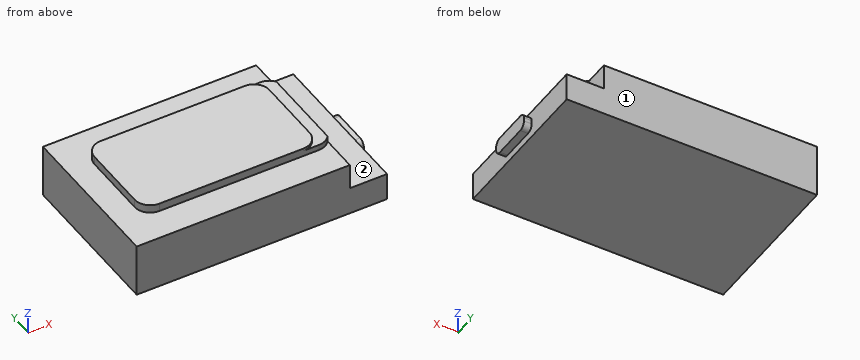
Solid Edge part; units mm, degrees
sketch "Sketch1" plane through (0, 0, 0) normal (0, 0, 1) x (1, 0, 0)
  line L0 (-25, -15.15) -> (25, -15.15)
  line L1 (25, -15.15) -> (25, 15.15)
  line L2 (25, 15.15) -> (-25, 15.15)
  line L3 (-25, 15.15) -> (-25, -15.15)
extrude "Protrusion1" add sketch "Sketch1" along normal blind 12
sketch "Sketch2" plane through (25, 0, 6) normal (1, 0, 0) x (0, 1, 0)
  line L0 (-0.65, -1.4) -> (2.65, -1.4)
  arc A0 (2.65, -1.4) -> (3.85, -2.6) centre (2.65, -2.6) cw
  line L1 (3.85, -2.6) -> (3.85, -3.3)
  arc A1 (2.65, -4.5) -> (3.85, -3.3) centre (2.65, -3.3) ccw
  line L2 (2.65, -4.5) -> (-3.95, -4.5)
  arc A2 (-5.15, -3.3) -> (-3.95, -4.5) centre (-3.95, -3.3) ccw
  line L3 (-5.15, -3.3) -> (-5.15, -2.6)
  arc A3 (-5.15, -2.6) -> (-3.95, -1.4) centre (-3.95, -2.6) cw
  line L4 (-3.95, -1.4) -> (-0.65, -1.4)
  line L5 (-15.15, -6) -> (15.15, -6)
  line L6 (15.15, -6) -> (15.15, 6)
  line L7 (15.15, 6) -> (-15.15, 6)
  line L8 (-15.15, 6) -> (-15.15, -6)
extrude "Wycięcie_1" cut sketch "Sketch2" against normal blind 1.5
sketch "Sketch3" plane through (-0.75, 0, 12) normal (0, 0, 1) x (1, 0, 0)
  line L0 (17.05, 15.15) -> (17.05, -15.15)
  line L1 (17.05, -15.15) -> (24.25, -15.15)
  line L2 (24.25, -15.15) -> (24.25, 15.15)
  line L3 (24.25, 15.15) -> (17.05, 15.15)
extrude "Wycięcie_2" cut sketch "Sketch3" against normal blind 6.6
sketch "Sketch4" plane through (-4.35, 0, 12) normal (0, 0, 1) x (1, 0, 0)
  line L0 (1.7674, -9.15) -> (-12.65, -9.15)
  arc A0 (-15.65, -6.15) -> (-12.65, -9.15) centre (-12.65, -6.15) ccw
  line L1 (-15.65, -6.15) -> (-15.65, 6.85)
  arc A1 (-15.65, 6.85) -> (-12.65, 9.85) centre (-12.65, 6.85) cw
  line L2 (-12.65, 9.85) -> (18.25, 9.85)
  arc A2 (18.25, 9.85) -> (21.25, 6.85) centre (18.25, 6.85) cw
  line L3 (21.25, 6.85) -> (21.25, -6.15)
  arc A3 (18.25, -9.15) -> (21.25, -6.15) centre (18.25, -6.15) ccw
  line L4 (18.25, -9.15) -> (1.7674, -9.15)
  line L5 (-28.1147, 19.5962) -> (36.8147, 19.5962)
  line L6 (36.8147, 19.5962) -> (36.8147, -19.5962)
  line L7 (36.8147, -19.5962) -> (-28.1147, -19.5962)
  line L8 (-28.1147, -19.5962) -> (-28.1147, 19.5962)
extrude "Wycięcie_3" cut sketch "Sketch4" against normal blind 1.6
sketch "Sketch5" plane through (-1.85, 0.35, 12) normal (0, 0, 1) x (1, 0, 0)
  line L0 (-18.15, 0) -> (-18.15, 6.5)
  arc A0 (-18.15, 6.5) -> (-15.15, 9.5) centre (-15.15, 6.5) cw
  line L1 (-15.15, 9.5) -> (12.75, 9.5)
  arc A1 (12.75, 9.5) -> (15.75, 6.5) centre (12.75, 6.5) cw
  line L2 (15.75, 6.5) -> (15.75, -6.5)
  arc A2 (15.75, -6.5) -> (12.75, -9.5) centre (12.75, -6.5) cw
  line L3 (-15.15, -9.5) -> (12.75, -9.5)
  arc A3 (-18.15, -6.5) -> (-15.15, -9.5) centre (-15.15, -6.5) ccw
  line L4 (-18.15, 0) -> (-18.15, -6.5)
  line L5 (-29.5576, 18.3934) -> (33.2576, 18.3934)
  line L6 (33.2576, 18.3934) -> (33.2576, -19.0934)
  line L7 (33.2576, -19.0934) -> (-29.5576, -19.0934)
  line L8 (-29.5576, -19.0934) -> (-29.5576, 18.3934)
extrude "Wycięcie_4" cut sketch "Sketch5" against normal blind 0.5
Source: CAD feature listing. Evaluate the final solid. Frame: model axes, mm. Face numbers are marked on the shaded views. A direction names the side the tool comes from. Coordinates: 2 decimals unless noted, no trailing zeros. Order: outer loops, then holes, each group sorted by start corner. A loop starts at its lowest first (then second) coordinate and runs counter-clockwise, first axis right, second up.
Item 1: Cut plane C-C (z = 6). Return loops of the section in (x, y), plus the area to 3 significant figures.
Output values:
outline: (-25, -15.15) - (16.3, -15.15) - (16.3, 15.15) - (-25, 15.15) - close
area: 1,250 mm2
Item 2: Material intervals for line 1 (Z direction, x = -13, y = -10.5); line 2 (Z direction, x = 18, y = -8); line 3 (X direction, y = 5.5, z = 5), sorted ascending.
Output values:
line 1: z = 0 to 10.4
line 2: z = 0 to 5.4
line 3: x = -25 to 23.5
Item 3: First-contact query: P1, Ø1, axis at y = -12, z = 10, coming from the +X side; P2, Ø0.8, axis at x = 24, z = 3, coming from the +Y side; P3, Ø0.8, axis at x = 24.5, y = -2, coming from the -Z side. Flat tips, straight axial feed; report the tip coordinate or a pass-through.
Output values:
P1: stops at x = 16.3
P2: stops at y = 3.85
P3: stops at z = 1.5
Item 4: Cut plane D-D (y = -11). Return loops of the section in (x, z), plus the area to 3 significant figures.
Output values:
outline: (-25, 0) - (23.5, 0) - (23.5, 5.4) - (16.3, 5.4) - (16.3, 10.4) - (-25, 10.4) - close
area: 468 mm2
Item 5: Cut plane A-A (y = 0.5). Return loops of the section in (x, z).
Output values:
outline: (-25, 0) - (23.5, 0) - (23.5, 1.5) - (25, 1.5) - (25, 4.6) - (23.5, 4.6) - (23.5, 5.4) - (16.3, 5.4) - (16.3, 11.5) - (13.9, 11.5) - (13.9, 12) - (-20, 12) - (-20, 10.4) - (-25, 10.4) - close
Item 6: Cut plane B-B (x = 1). Return loops of the section in (y, z).
Output values:
outline: (-15.15, 0) - (15.15, 0) - (15.15, 10.4) - (9.85, 10.4) - (9.85, 12) - (-9.15, 12) - (-9.15, 10.4) - (-15.15, 10.4) - close
Item 7: Set-up query: the marked faces 1 and 2. Return all of +Z, -Z, +X, -X, +Y, -Y with unobstructed straight access to the full face (end or side cutting, diameter ignored); none if empty.
Output values:
face 1: +Z, -Z, +X, -X, +Y
face 2: +Z, +X, +Y, -Y
